```python
from build123d import *

# Parameters (mm, degrees)
F0_R          = 15.875
F1_DEPTH      = 31.75
F2_R          = 6.35
F3_DEPTH      = 44.45
F5_DEPTH      = 76.2
F5_DEPTH_BACK = 76.2


with BuildPart() as f1:
    # F0 (on Top) → F1 (new body)
    with BuildSketch(Plane.XY):
        Circle(F0_R)
    extrude(amount=F1_DEPTH)

    # F2 (on face) → F3 (join)
    with BuildSketch(Plane(origin=(0, 0, 0), x_dir=(1, 0, 0), z_dir=(0, 0, -1))):
        Circle(F2_R)
    extrude(amount=F3_DEPTH)

    # F4 (on Right) → F5 (join, two sides)
    with BuildSketch(Plane.YZ) as f5_sk:
        with BuildLine():
            ThreePointArc((0, 20.32), (-4.445, 15.875), (0, 11.43))
            Line((0, 11.43), (0, 20.32))
        make_face()
        with BuildLine():
            Line((0, 20.32), (0, 11.43))
            ThreePointArc((0, 11.43), (3.14309, 12.73191), (4.445, 15.875))
            ThreePointArc((4.445, 15.875), (3.14309, 19.01809), (0, 20.32))
        make_face()
    extrude(amount=F5_DEPTH)
    extrude(f5_sk.sketch, amount=-F5_DEPTH_BACK)

    # F6 (on Front) → F7 (revolve)
    with BuildSketch(Plane.XZ):
        with BuildLine():
            ThreePointArc((95.496059, 15.875), (87.616765, 25.775706), (76.2, 20.32))
            Line((76.2, 20.32), (76.2, 15.875))
            Line((76.2, 15.875), (95.496059, 15.875))
        make_face()
        with BuildLine():
            Line((-76.2, 15.875), (-76.2, 20.32))
            ThreePointArc((-76.2, 20.32), (-87.616765, 25.775706), (-95.496059, 15.875))
            Line((-95.496059, 15.875), (-76.2, 15.875))
        make_face()
    revolve(axis=Axis((48.289891, 0, 15.875), (1, 0, 0)))


solid = f1.part
```
Input: part model. Units: mm. Frame: model coordinates. Coordinates: 2 decimals unless noted, no trailing zeros. Write each loop counter-clockwise with the first axis right and the second up, starting at its lowest first coordinate (ties: lowest second). Pieces come first, ordered by that corner, then holes.
1) Section B-B on z = -9. Output: boundary loops of the cut face in (x, y), and give its area (3 significant figures).
2) Material intervals for line 1 along X through (y, z) = (0, -35); line 2 along Z through (x, y) = (8, -9.5); line 3 along Z through (x, y) = (50, -3.5), sorted ascending.
3) Mould query, pull axis X, two halves, no side actions, for faces 1 (the cylindrical face through (14.664, -6.08, 15.653)), 2 (the cylindrical face through (-1.38, 6.2, -21.91)), 3 (the flat face through (7, 0, 0)). Classes: pulls with the +X half, pulls with the -X half, needs draft (parallel to the pull), parting line crosses it, or undercut.
4) Section A-A on x = 0. Output: boundary loops of the cut face in (y, z) (3 decimals).
5) Pin query (flat end, axial travel): pin 1 Ø1.5 at (x, z) = (7, 5.5) entering from +Y; pin 2 Ø2 at (x, y) = (-39.5, -5) entering from -Z; pin 3 Ø12 at (x, y) = (17, 7) entering from -Z; pin 4 Ø5 at (y, z) = (9.5, -18.5) entering from +X. Return the tip coordinate at first contact, or that it passes through.
6) Section C-C on x = 70. Output: boundary loops of the cut face in (y, z) (3 decimals), and give its area (3 significant figures).
Check result:
1. outline: circle Ø12.7 at (0, 0)
1. area: 127 mm2
2. line 1: x = -6.35 to 6.35
2. line 2: z = 0 to 31.75
2. line 3: z = 13.13 to 18.62
3. face 1: undercut
3. face 2: parting line crosses it
3. face 3: needs draft
4. outline: (-15.875, 0) - (-6.35, 0) - (-6.35, -44.45) - (6.35, -44.45) - (6.35, 0) - (15.875, 0) - (15.875, 31.75) - (-15.875, 31.75) - close
5. pin 1: stops at y = 14.59
5. pin 2: stops at z = 13.94
5. pin 3: stops at z = 0
5. pin 4: passes through
6. outline: (0, 11.43) arc R4.445 ccw to (4.445, 15.875) arc R4.445 ccw to (0, 20.32) arc R4.445 ccw to start
6. area: 62.1 mm2
